Verification items for this drawing (mm, ordinates from the low corner). A direction names the side the tool comes from. Coordinates: 2 decimals unless noted, no trailing zeros. Order: outer loops, then holes, each group sorted by start corner. A loop starts at its lowest first (then second) coordinate and runs counter-clockwise, first axis right, second up. Notation, with made-up numbers: (41, 34.25) -> (51, 34.25) arc R4 ccw to (51, 39.25) -> close; hole circle Ø3 at (-22.75, 83). An arc over 180 degrees is marked (long way). Write each question's results on one line, items separated by ' | '. Start each with the question number.
(1) Cross-section at C-C on z = 4. Enter the section's corners in (x, y).
(2) Cross-section at A-A on z = 3. Enter the section's corners in (x, y).
(3) Thickness scan on probe 1 along Z at (x, y) = (10, 8.05); probe 2 along X at (y, z) = (8.45, 3); probe 3 along Y at (x, z) = (16.5, 2.9). Record the ranges inside material, lowest first. Write a range as [from, to].
(4) Set-up check for the marked faces 4, 5, 6 and 7: record each of +Z, -Z, +X, -X, +Y, -Y from which the full face is reachable in a straight line by a thin tool's end or side.
(5) Draft check along Y on the marked faces 1, 2 and 3. Enter one of: +Y half, -Y half, draft (parallel to the pull), parting line (faces both ways), or undercut.
(6) Cross-section at D-D on x = 4.75. Enter the section's corners in (y, z), and give its area (3 significant figures).
(7) Cross-section at B-B on y = 5.25. Enter the section's corners in (x, z).
(8) Go/stop test with flat-tipped pins: pin 1 (6 mm diameter, centred on x = 13, y = 7.5, fed in from +Z); pin 2 (1.5 mm diameter, centred on x = 7, y = 6.5, fed in from -Z). Record where each tip stops, or that it passes through.
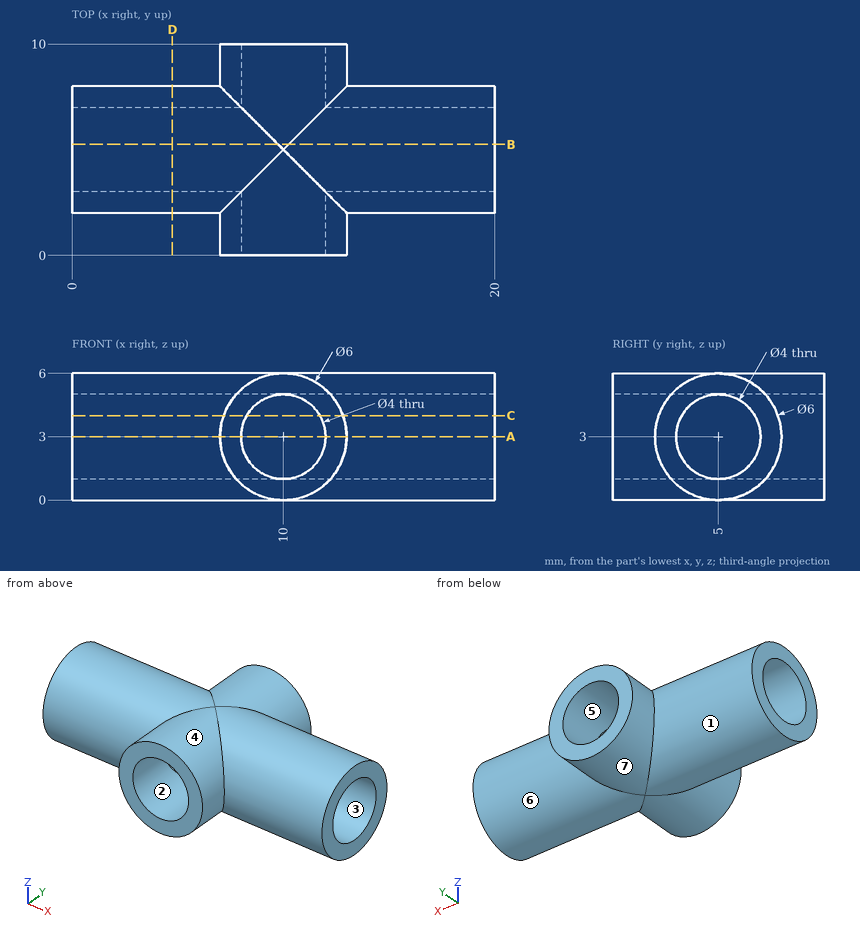
Results are:
1) outline: (0, 2.17) -> (7.17, 2.17) -> (7.17, 0) -> (8.27, 0) -> (8.27, 3.27) -> (0, 3.27) -> close; (0, 6.73) -> (8.27, 6.73) -> (8.27, 10) -> (7.17, 10) -> (7.17, 7.83) -> (0, 7.83) -> close; (11.73, 0) -> (12.83, 0) -> (12.83, 2.17) -> (20, 2.17) -> (20, 3.27) -> (11.73, 3.27) -> close; (11.73, 6.73) -> (20, 6.73) -> (20, 7.83) -> (12.83, 7.83) -> (12.83, 10) -> (11.73, 10) -> close
2) outline: (0, 2) -> (7, 2) -> (7, 0) -> (8, 0) -> (8, 3) -> (0, 3) -> close; (0, 7) -> (8, 7) -> (8, 10) -> (7, 10) -> (7, 8) -> (0, 8) -> close; (12, 0) -> (13, 0) -> (13, 2) -> (20, 2) -> (20, 3) -> (12, 3) -> close; (12, 7) -> (20, 7) -> (20, 8) -> (13, 8) -> (13, 10) -> (12, 10) -> close
3) probe 1: z = [0, 1], [5, 6] | probe 2: x = [7, 8], [12, 13] | probe 3: y = [2, 3], [7, 8]
4) face 4: -Y | face 5: +Y, -Y | face 6: +X | face 7: +Y
5) face 1: parting line | face 2: draft | face 3: undercut
6) outline: circle Ø6 at (5, 3); hole circle Ø4 at (5, 3) | area: 15.7 mm2
7) outline: (0, 0.01) -> (9.75, 0.01) arc R3 ccw to (10.25, 0.01) -> (20, 0.01) -> (20, 1.02) -> (10.25, 1.02) arc R2 cw to (9.75, 1.02) -> (0, 1.02) -> close; (0, 4.98) -> (9.75, 4.98) arc R2 cw to (10.25, 4.98) -> (20, 4.98) -> (20, 5.99) -> (10.25, 5.99) arc R3 ccw to (9.75, 5.99) -> (0, 5.99) -> close
8) pin 1: stops at z = 6 | pin 2: stops at z = 0.1
